For this review, use the dimensioned drawing (mm, ordinates from the lowest corner) and the shaded views. Coordinates: 2 decimals unless noted, no trailing zeros. Write each loop counter-clockwise with the first axis right and the second up, starting at its lowest first coordinate (ties: lowest second). Pieces come first, ordered by that corner, then holes. Notation, with made-up numbers: M 88,-9.5 L 126,-9.5 A27 cw 126,20.5 Z; hole C -32.75,61.25 d5. An arc over 180 degrees is marked long. Return JSON: item names as keys, results as strings.
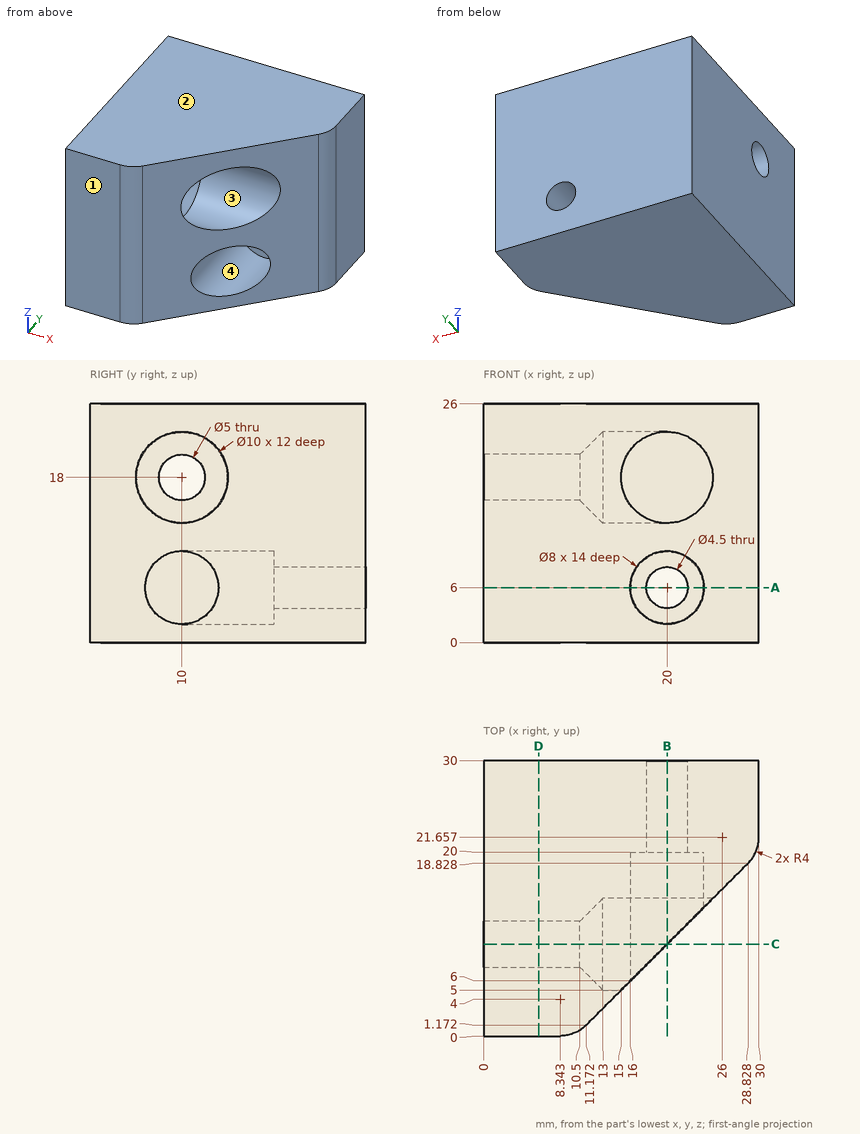
1. We need section B-B (x = 20). State the section outline as (y, z) points.
Checks:
{"outline": "M 10,0 L 30,0 L 30,3.75 L 20,3.75 L 20,2 L 10,2 Z; M 10,10 L 20,10 L 20,8.25 L 30,8.25 L 30,26 L 10,26 L 10,23 A5 cw 10,13 Z"}
2. Draft analysis for pull direction Z (two halves, no side actions). For the marked faces 1, 2, 3 and 4, state which applies: +Z half, -Z half, draft (parallel to the pull), parting line (faces both ways), or undercut.
Checks:
{"face 1": "draft", "face 2": "+Z half", "face 3": "undercut", "face 4": "undercut"}
3. Clearance check with flat-ended pins moving along their axes: pin 1 Ø8 at (y, z) = (15, 16.5) entering from +X; pin 2 Ø10 at (x, z) = (19.5, 16.5) entering from -Y; pin 3 Ø3 at (y, z) = (9.5, 20.5) entering from +X; pin 4 Ø1 at (y, z) = (9, 21.5) entering from -X. State where each tip first meets the part, or that it passes through.
Checks:
{"pin 1": "x = 28.99", "pin 2": "y = 4.5", "pin 3": "x = 12.05", "pin 4": "x = 0"}
4. Wall thickness on L1, parallel to Z at x = 7.25, y = 10; L2, parallel to Z at x = 18, y = 10 (1 decimal); L3, parallel to Z at x = 20, y = 22.75: over which ranges is each line inside the solid? List them lowest first. Write a range as from..to.
Checks:
{"L1": "0..15.5, 20.5..26", "L2": "0..2.5, 9.5..13, 23..26", "L3": "0..3.75, 8.25..26"}
5. We need section C-C (y = 10). State the section outline as (x, z) points.
Checks:
{"outline": "M 0,0 L 20,0 L 20,2 A4 cw 20,10 L 20,13 L 13,13 L 10.5,15.5 L 0,15.5 Z; M 0,20.5 L 10.5,20.5 L 13,23 L 20,23 L 20,26 L 0,26 Z"}
6. We need section D-D (x = 6). State the section outline as (y, z) points, plus the area to 3 significant figures.
Checks:
{"outline": "M 0,0 L 30,0 L 30,26 L 0,26 Z; hole C 10,18 d5", "area": "760 mm2"}
7. We need section A-A (z = 6). State the section outline as (x, y) points, plus the area to 3 significant figures.
Checks:
{"outline": "M 0,0 L 8.34,0 A4 ccw 11.17,1.17 L 16,6 L 16,20 L 17.75,20 L 17.75,30 L 0,30 Z; M 22.25,20 L 24,20 L 24,14 L 28.83,18.83 A4 ccw 30,21.66 L 30,30 L 22.25,30 Z", "area": "574 mm2"}
